Job drawing, mm, ordinate dimensions from the low corner. One solid piece. Coordinates: 2 decimals unless noted, no trailing zeros. Loops run counter-clockwise (first coordinate to the right, second up) from the corner with the lowest first, then second, coordinate; pieces in that order, holes last. Notation, with made-up numbers: M 51,-3.75 L 104,-3.75 A32 ccw 104,25.25 Z; hole C 10,55.5 d2. An arc over 180 degrees is marked long. Answer as a JSON object with one key per item and string values. Group by question number.
1. Drill centre lines: L1, parallel to Y at x = 154, z = 0.75; L2, parallel to X at y = 14, z = 1.95. Where is each one in solid material? Low to high.
2. Saw through at C-C on z = 1.05. Write the cut outline in (x, y), then the cut area to 3 significant figures.
3. Saw through at B-B on x = 34. Write the cut outline in (y, z).
4. Saw through at A-A on y = 72. Write the cut outline in (x, z).
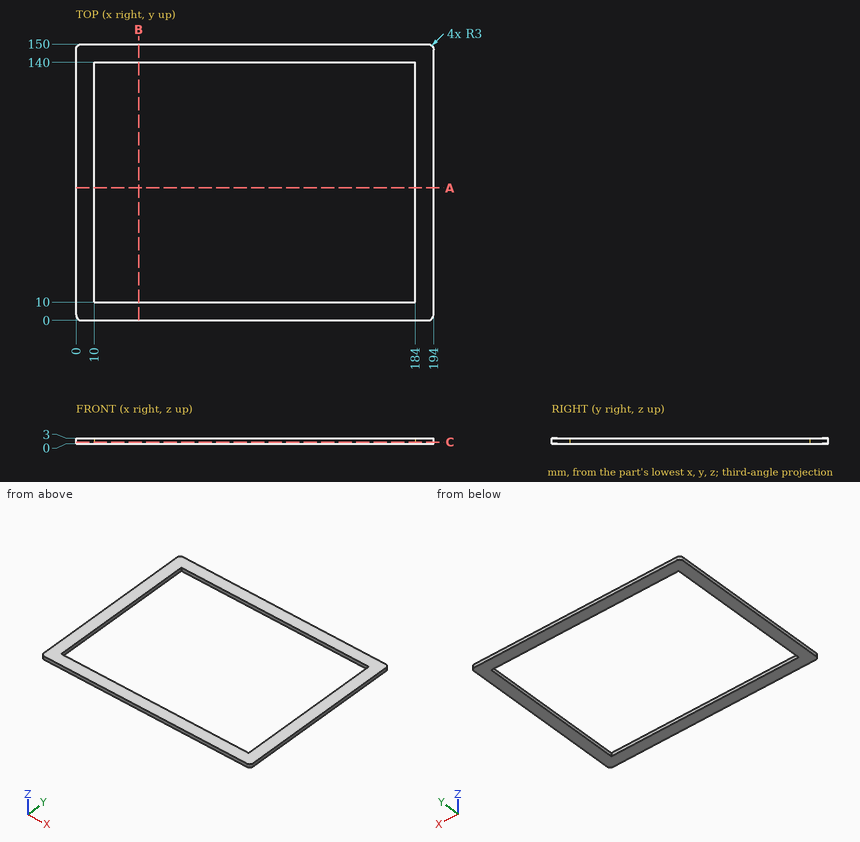
Outcome:
{
 "1": {"L1": "y = 0 to 10, 140 to 150", "L2": "x = 0 to 10, 184 to 194"},
 "2": {"outline": "M 0,3 A3 ccw 3,0 L 191,0 A3 ccw 194,3 L 194,147 A3 ccw 191,150 L 3,150 A3 ccw 0,147 Z; hole M 10,10 L 184,10 L 184,140 L 10,140 Z", "area": "6,470 mm²"},
 "3": {"outline": "M 0,0 L 10,0 L 10,3 L 0,3 Z; M 140,0 L 150,0 L 150,3 L 140,3 Z"},
 "4": {"outline": "M 0,0 L 10,0 L 10,3 L 0,3 Z; M 184,0 L 194,0 L 194,3 L 184,3 Z"}
}
